Input: dimensioned drawing with shaded views. Units: mm. Origin: part minimum x, y, z. A direction names the side the tool comes from. Round coordinates to 2 decimals unless told otherwise and drop trailing zeros. Loops run counter-clockwise (first coordinate to the right, second up) from the corner with the lowest first, then second, coordinate; pieces in that order, holes last. Notation, with made-up numbers: (-7.5, 6) - (38.5, 6) arc R20 ccw to (38.5, 15) - close; hole circle Ø4 at (23.5, -1). An arc over 180 degrees is marked (long way). Answer as a JSON object with one key per item and string values. Group by question number.
Item 1: Section C-C (z = 10). Return the cut outline in (x, y), plus the area to 3 significant figures.
Item 2: Section A-A (y = 252). Return the cut outline in (x, z) (1 decimal).
Item 3: Line query: line 1 (Z direction, x = 436.5, y = 219); line 2 (Y direction, x = 148.5, z = 2); line 3 (Y direction, x = 455.5, z = 19.5). Output: solid intervals per line, ascending.
Item 4: Section D-D (y = 83). Return the cut outline in (x, z).
Item 5: Section B-B (x = 463). Return the cut outline in (y, z).
Item 6: Reachability of the marked faces 1 and 2 from +Z, -Z, +X, -X, +Y, -Y: full face, straight path, thin tool, end or side. Return the list, or none.
Item 7: First-contact query: pin 1 (1.5 mm diameter, centred on x = 68.5, z = 3.5, fed in from -Y); pin 2 (1 mm diameter, centred on x = 142.5, y = 212, fed in from +Z); pin 3 (2.5 mm diameter, centred on y = 58.5, z = 2, fed in from -X). Flat tips, straight axial feed; report the tip coordinate or a pass-through.
Item 8: Draft query along X for the marked faces 3 and 4. Return one class per face: released by +X, released by -X, zero draft, split by the parting line, or undercut.
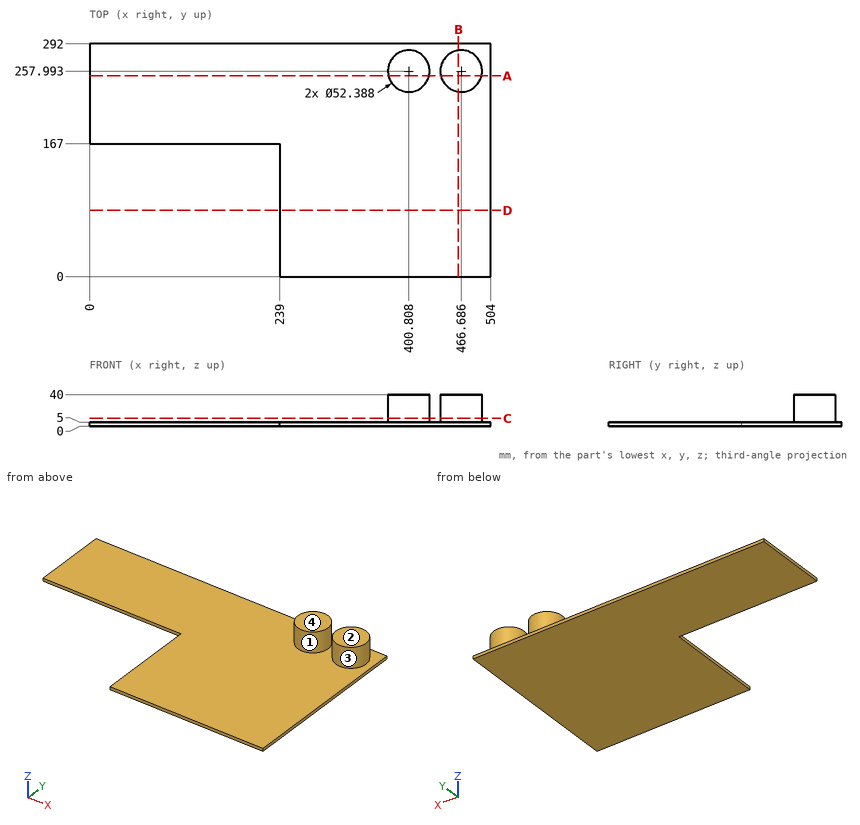
Values:
{
 "1": {"outline": "circle Ø52.39 at (400.81, 257.99); circle Ø52.39 at (466.69, 257.99)", "area": "4,310 mm^2"},
 "2": {"outline": "(0, 0) - (504, 0) - (504, 5) - (492.2, 5) - (492.2, 40) - (441.2, 40) - (441.2, 5) - (426.3, 5) - (426.3, 40) - (375.3, 40) - (375.3, 5) - (0, 5) - close"},
 "3": {"line 1": "z = 0 to 5", "line 2": "y = 167 to 292", "line 3": "y = 234.31 to 281.68"},
 "4": {"outline": "(239, 0) - (504, 0) - (504, 5) - (239, 5) - close"},
 "5": {"outline": "(0, 0) - (292, 0) - (292, 5) - (283.93, 5) - (283.93, 40) - (232.06, 40) - (232.06, 5) - (0, 5) - close"},
 "6": {"face 1": "+Z", "face 2": "+Z, +X, -X, +Y, -Y"},
 "7": {"pin 1": "stops at y = 167", "pin 2": "stops at z = 5", "pin 3": "stops at x = 239"},
 "8": {"face 3": "undercut", "face 4": "zero draft"}
}
